from build123d import *

# Parameters (mm, degrees)
EXTRUDE_1_DEPTH      = 8
SKETCH_2_R           = 2
EXTRUDE_2_DEPTH      = 1
EXTRUDE_3_DEPTH      = 0.2
EXTRUDE_3_DEPTH_BACK = 1
SKETCH_3_R           = 2
EXTRUDE_4_DEPTH      = 2.5
EXTRUDE_5_DEPTH      = 3
CHAMFER_1_SIZE       = 1
CUT_EXTRUDE_1_DEPTH  = 0.2


with BuildPart() as part:
    # 草图1 → 凸台-拉伸1 (new body)
    with BuildSketch(Plane(origin=(0, 0, 0), x_dir=(1, 0, 0), z_dir=(0, 1, 0))):
        with BuildLine():
            Line((0.9, 0.9), (0.9, -0.9))
            ThreePointArc((0.9, -0.9), (0, -1.8), (-0.9, -0.9))
            Line((-0.9, -0.9), (-0.9, 0.9))
            ThreePointArc((-0.9, 0.9), (0, 1.8), (0.9, 0.9))
        make_face()
    extrude(amount=EXTRUDE_1_DEPTH)

    # 草图2 → 凸台-拉伸2 (add)
    with BuildSketch(Plane(origin=(0, 8, 0), x_dir=(1, 0, 0), z_dir=(0, 1, 0))):
        with Locations(Location((0, 0, 0), (0, 0, 270))):
            Circle(SKETCH_2_R)
    extrude(amount=-EXTRUDE_2_DEPTH)

    # 草图3 → 凸台-拉伸3 (add, two sides: drawn at the far end of the back side and taken through both)
    with BuildSketch(Plane.XZ.offset(-EXTRUDE_3_DEPTH_BACK)):
        with Locations(Location((0, 0, 0), (0, 0, 90))):
            Circle(SKETCH_3_R)
    extrude(amount=EXTRUDE_3_DEPTH + EXTRUDE_3_DEPTH_BACK)

    # 草图6 → 凸台-拉伸4 (add)
    with BuildSketch(Plane(origin=(0, 8, 0), x_dir=(1, 0, 0), z_dir=(0, 1, 0))):
        with BuildLine():
            Line((-0.9, -0.9), (-0.9, 0.9))
            ThreePointArc((-0.9, 0.9), (0, 1.8), (0.9, 0.9))
            Line((0.9, 0.9), (0.9, -0.9))
            ThreePointArc((0.9, -0.9), (0, -1.8), (-0.9, -0.9))
        make_face()
    extrude(amount=EXTRUDE_4_DEPTH)

    # 草图7 → 凸台-拉伸5 (add)
    with BuildSketch(Plane(origin=(0, 10.5, 0), x_dir=(1, 0, 0), z_dir=(0, 1, 0))):
        with BuildLine():
            Line((-5, -3), (-5, 1))
            ThreePointArc((-5, 1), (-4.707106781, 1.707106781), (-4, 2))
            Line((-4, 2), (4, 2))
            ThreePointArc((4, 2), (4.707106781, 1.707106781), (5, 1))
            Line((5, 1), (5, -3))
            ThreePointArc((5, -3), (0, -8), (-5, -3))
        make_face()
    extrude(amount=EXTRUDE_5_DEPTH)

    # 倒角1
    chamfer_1_edges = [part.edges().sort_by_distance(p)[0] for p in [
        (4.707106781, 13.5, -1.707106781),
        (0, 13.5, -2),
        (-4.707106781, 13.5, -1.707106781),
        (-5, 13.5, 1),
        (0, 13.5, 8),
        (5, 13.5, 1),
    ]]
    chamfer(chamfer_1_edges, length=CHAMFER_1_SIZE - 0.0001)  # a hair under: the kernel refuses the full size

    # 草图8 → 切除-拉伸1 (cut)
    with BuildSketch(Plane.XZ.offset(0.2)):
        with BuildLine():
            Line((-0.4, 1.2), (0.4, 1.2))
            ThreePointArc((0.4, 1.2), (1.6, 0), (0.4, -1.2))
            Line((0.4, -1.2), (-0.4, -1.2))
            ThreePointArc((-0.4, -1.2), (-1.6, 0), (-0.4, 1.2))
        make_face()
    extrude(amount=-CUT_EXTRUDE_1_DEPTH, mode=Mode.SUBTRACT)


solid = part.part
Geometry: final body of the model. Coordinates: model frame, mm. A direction names the side the tool comes from. Coordinates: 2 decimals unless noted, no trailing zeros. Order: outer loops, then holes, each group sorted by start corner. A loop starts at its lowest first (then second) coordinate and runs counter-clockwise, first axis right, second up. Notation, with made-up numbers: M 73.5,11.5 L 83.5,11.5 A24 ccw 83.5,32.5 Z; hole C 40.5,-36.75 d5. An arc over 180 degrees is marked long. One line per question, with ' | ' between items. Start each with the question number.
Item 1: Pin query (flat end, axial travel): pin 1 Ø0.7 at (x, z) = (-0.5, 0.5) entering from -Y; pin 2 Ø1.4 at (y, z) = (3.5, 0) entering from -X; pin 3 Ø5 at (x, z) = (-3, 3.5) entering from -Y. Return the tip coordinate at first contact, or that it passes through.
Item 2: Draft query along Y for faces 6 (the flat face through (1.4, 8, 0)), 7 (the conical face through (4.355, 12.993, -1.362)), 8 (the cylindrical face through (4.699, 11.486, -1.715)). Return one class per face: released by +Y, released by -Y, zero draft, split by the parting line, or undercut.
Item 3: Cut plane A-A, the plane x = 0. Return the cut outline in (y, z), then the cut area to 3 significant figures.
Item 4: Cut plane C-C, the plane y = 11. Return the cut outline in (x, z), then the cut area to 3 significant figures.
Item 5: Cut plane B-B, the plane z = 0. Return the cut outline in (x, y).
Item 6: Cut plane D-D, the plane z = 2.25. Return the cut outline in (x, y).
Item 7: Ray query, probe 1 along Y at (x, z) = (1.25, 4); probe 2 along X at (y, z) = (13.25, 6.75); probe 3 along X at (y, z) = (4.5, 0.5). Return the intervals inside material, ascending. Write a range as [from, to].
Item 8: Set-up query: faces 1 (the flat face through (0, 0, 0)), 2 (the flat face through (-0.9, 4, 0)), 3 (the cylindrical face through (0, 9.2, -1.8)), 4 (the cylindrical face through (0, 9.2, 1.8)), 5 (the flat face through (0.9, 4, 0)). Return all of +Z, -Z, +X, -X, +Y, -Y with unobstructed straight access to the full face (end or side cutting, diameter ignored); none if empty.
A:
1) pin 1: stops at y = 0 | pin 2: stops at x = -0.9 | pin 3: stops at y = 10.5
2) face 6: undercut | face 7: released by +Y | face 8: zero draft
3) outline: M -0.2,-2 L 1,-2 L 1,-1.8 L 7,-1.8 L 7,-2 L 8,-2 L 8,-1.8 L 10.5,-1.8 L 10.5,-2 L 12.5,-2 L 13.5,-1 L 13.5,7 L 12.5,8 L 10.5,8 L 10.5,1.8 L 8,1.8 L 8,2 L 7,2 L 7,1.8 L 1,1.8 L 1,2 L -0.2,2 L -0.2,1.2 L 0,1.2 L 0,-1.2 L -0.2,-1.2 Z | area: 67.9 mm2
4) outline: M -5,-1 A1 ccw -4,-2 L 4,-2 A1 ccw 5,-1 L 5,3 A5 ccw -5,3 Z | area: 88.8 mm2
5) outline: M -5,10.5 L -0.9,10.5 L -0.9,8 L -2,8 L -2,7 L -0.9,7 L -0.9,1 L -2,1 L -2,-0.2 L -1.6,-0.2 L -1.6,0 L 1.6,0 L 1.6,-0.2 L 2,-0.2 L 2,1 L 0.9,1 L 0.9,7 L 2,7 L 2,8 L 0.9,8 L 0.9,10.5 L 5,10.5 L 5,12.5 L 4,13.5 L -4,13.5 L -5,12.5 Z
6) outline: M -5,10.5 L 5,10.5 L 5,12.5 L 4,13.5 L -4,13.5 L -5,12.5 Z
7) probe 1: y = [10.5, 13.5] | probe 2: x = [-2, 2] | probe 3: x = [-0.9, 0.9]
8) face 1: -Y | face 2: +Z, -Z, -X | face 3: -Z | face 4: +Z | face 5: +Z, -Z, +X
